Here's how the part is built. I have some questions about the finished solid (model axes, mm). Give positions to 0.01 mm unless a question says otherwise; leave off trailing zeros. Loops run counter-clockwise (first coordinate to the right, second up) from the corner with the lowest first, then second, coordinate; pieces in that order, holes last. Notation, with made-up numbers: (-13, 2.5) - (36, 2.5) arc R14 cw to (36, 11.5) - close; hole circle Ø4 at (26, -33). An arc over 180 degrees is marked (long way). Use a Markdown table: item, result.
from build123d import *

# Parameters (mm, degrees)
F0_W     = 65
F0_H     = 132
F1_DEPTH = 8.9
F2_R     = 5
F3_R     = 4
F4_SIZE  = 2
F6_W     = 55
F6_H     = 100
F7_DEPTH = 0.01
F8_W     = 10
F8_H     = 2
F9_DEPTH = 1


with BuildPart() as f1:
    # F0 (on Front) → F1 (new body)
    with BuildSketch(Plane.XZ):
        Rectangle(F0_W, F0_H)
    extrude(amount=F1_DEPTH)

    # F2
    f2_edges = [f1.edges().sort_by_distance(p)[0] for p in [
        (-32.5, -4.45, 66),
        (32.5, -4.45, 66),
        (32.5, -4.45, -66),
        (-32.5, -4.45, -66),
    ]]
    fillet(f2_edges, radius=F2_R)

    # F3
    f3_edges = [f1.edges().sort_by_distance(p)[0] for p in [
        (32.5, 0, 0),
    ]]
    fillet(f3_edges, radius=F3_R)

    # F4
    f4_edges = [f1.edges().sort_by_distance(p)[0] for p in [
        (32.5, -8.9, 0),
    ]]
    chamfer(f4_edges, length=F4_SIZE)

    # F6 (on face) → F7 (cut)
    with BuildSketch(Plane.XZ.offset(8.9)):
        Rectangle(F6_W, F6_H)
    extrude(amount=-F7_DEPTH, mode=Mode.SUBTRACT)

    # F8 (on face) → F9 (cut)
    with BuildSketch(Plane.XZ.offset(8.9)):
        with Locations((0, 57)):
            Rectangle(F8_W, F8_H)
    extrude(amount=-F9_DEPTH, mode=Mode.SUBTRACT)


solid = f1.part
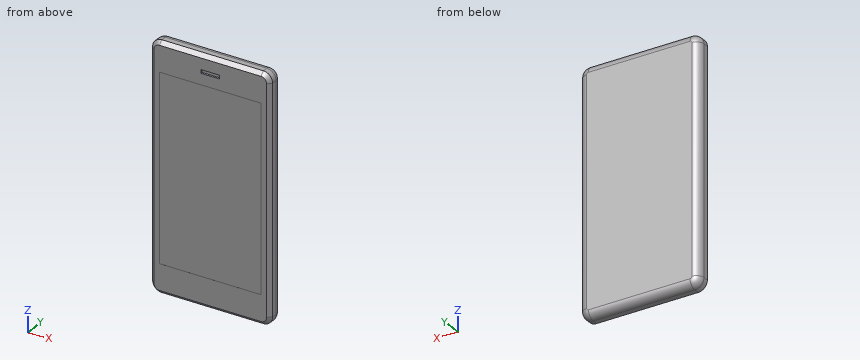
(1) Will these pins go through, and if not, where does the flat tip stop? pin 1 (0.5 mm diameter, centred on x = 2.5, y = -8.5, fed in from +Z); pin 2 (1.1 mm diameter, centred on y = -8, z = 57, fed in from +X); pin 3 (1.5 mm diameter, centred on x = 3, z = -44, fed in from -Y).
A:
| item | result |
|---|---|
| pin 1 | z = 64.65 |
| pin 2 | x = 31.95 |
| pin 3 | y = -8.89 |
(2) Suppose I cut it at B-B on z = -57.5. Write out the boundary of the cut face in (x, y), plus the area to 3 significant figures.
A:
| item | result |
|---|---|
| outline | (-32.5, -6.9) - (-30.5, -8.9) - (30.5, -8.9) - (32.5, -6.9) - (32.5, -4) arc R4 ccw to (28.5, 0) - (-28.5, 0) arc R4 ccw to (-32.5, -4) - close |
| area | 568 mm2 |
(3) If I drill on line 1 (Y direction, x = -15, z = -24); line 2 (Z direction, x = 26, y = -3); line 3 (Z direction, x = 7.5, y = -8), over which ranges is the centre line in solid material (lowest first)?
A:
| item | result |
|---|---|
| line 1 | -8.89 to 0 |
| line 2 | -65.87 to 65.87 |
| line 3 | -64.9 to 64.9 |
